Read the model definition and answer for the solid it produces. Units are mm, in the model's axes. Face numbers are marked on the shaded views. Coordinates: 2 decimals unless noted, no trailing zeros. Write each loop counter-clockwise with the first axis right and the second up, starting at its lowest first coordinate (ties: lowest second). Pieces come first, ordered by that corner, then holes. Notation, with made-up numbers: (59, -15) -> (100, -15) arc R29 ccw to (100, 22) -> close; hole circle Ø2 at (-34.75, 73.5). An arc over 180 degrees is marked (long way). Answer as a JSON object with one key per item and string values. Group by question number.
(1) Find section D-D (x = 1.7). Give the vertices of the cut face in (y, z).
(2) For a pull along X with two mould halves and no side action, classify the marked faces 1, 2 and 3 as +X half, -X half, draft (parallel to the pull), parting line (faces both ways), or undercut.
(3) Find section C-C (y = -0.8). Give the vertices of the cut face in (x, z), then the cut area to 3 significant figures.
(4) Find section A-A (x = 0). Give the vertices of the cut face in (y, z).
(5) Find section B-B (z = 1.25). Give the vertices of the cut face in (x, y).
(6) Straight lines are drawn through the part: L1, parallel to Y at x = 0, z = -0.25; L2, parallel to Y at x = 1.1, z = -6.75; L3, parallel to X at y = -0.7, z = 8.75. For each, find the intervals that lie inside material, in ascending order.
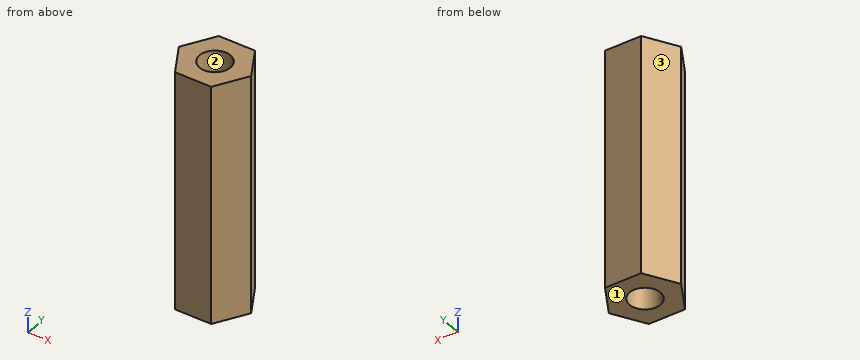
Autodesk Inventor part; units mm, degrees
ref_plane "YZ Plane" through (0, 0, 0) normal (1, 0, 0) x (0, 1, 0)
ref_plane "XZ Plane" through (0, 0, 0) normal (0, 1, 0) x (-1, 0, 0)
ref_plane "XY Plane" through (0, 0, 0) normal (0, 0, 1) x (1, 0, 0)
sketch "Skizze2" plane through (0, 0, 0) normal (0, 0, 1) x (1, 0, 0)
  line L0 (-1.4434, 2.5) -> (1.4434, 2.5)
  line L1 (1.4434, 2.5) -> (2.8868, 0)
  line L2 (2.8868, 0) -> (1.4434, -2.5)
  line L3 (1.4434, -2.5) -> (-1.4434, -2.5)
  line L4 (-1.4434, -2.5) -> (-2.8868, 0)
  line L5 (-2.8868, 0) -> (-1.4434, 2.5)
  line L6 (-1.4434, 2.5) -> (1.4434, -2.5) construction
  point P0 (0, 0)
  point P1 (0, 0)
  dimension "d17" = 120
  dimension "d19" = 120
  dimension "d22" = 120
  dimension "d36" = 5
extrude "Extrusion1" add sketch "Skizze2" along normal mid plane 19
sketch "Skizze4" plane through (0, 0, 9.5) normal (0, 0, 1) x (1, 0, 0)
  point P0 (0, 0)
hole "Bohrung1" at (0, 0, 9.5) direction (0, 0, -1) diameter 2.459 end through all
properties part number "Abstandshalter_M3"
Results below:
{
 "1": {"outline": "(-2.06, -9.5) -> (2.06, -9.5) -> (2.06, 9.5) -> (-2.06, 9.5) -> close"},
 "2": {"face 1": "draft", "face 2": "undercut", "face 3": "-X half"},
 "3": {"outline": "(-2.42, -9.5) -> (-0.93, -9.5) -> (-0.93, 9.5) -> (-2.42, 9.5) -> close; (0.93, -9.5) -> (2.42, -9.5) -> (2.42, 9.5) -> (0.93, 9.5) -> close", "area": "56.7 mm2"},
 "4": {"outline": "(-2.5, -9.5) -> (-1.23, -9.5) -> (-1.23, 9.5) -> (-2.5, 9.5) -> close; (1.23, -9.5) -> (2.5, -9.5) -> (2.5, 9.5) -> (1.23, 9.5) -> close"},
 "5": {"outline": "(-2.89, 0) -> (-1.44, -2.5) -> (1.44, -2.5) -> (2.89, 0) -> (1.44, 2.5) -> (-1.44, 2.5) -> close; hole circle Ø2.46 at (0, 0)"},
 "6": {"L1": "y = -2.5 to -1.23, 1.23 to 2.5", "L2": "y = -2.5 to -0.55, 0.55 to 2.5", "L3": "x = -2.48 to -1.01, 1.01 to 2.48"}
}
